Geometry: final body of the model. Coordinates: model frame, mm. Give positions to 0.01 mm unless a question says otherwise; leave off trailing zeros.
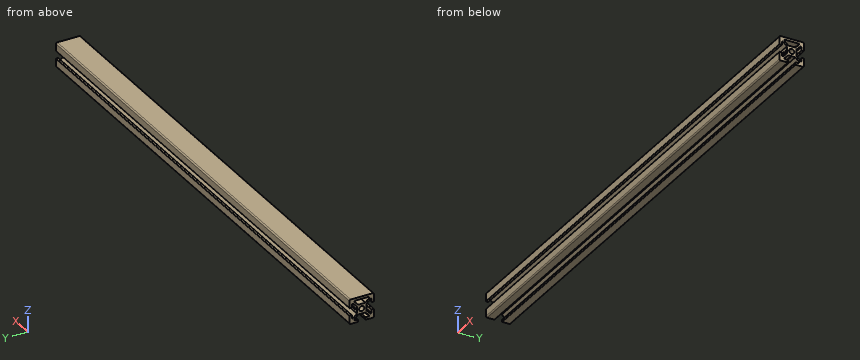
from build123d import *

# Parameters (mm, degrees)
F1_DEPTH = 210


# Not quite as in the source:
# - ends of sketch curves that miss each other by under 0.0002 mm in the source are joined


with BuildPart() as f1:
    # F0 (on Right) → F1 (new body, symmetric)
    with BuildSketch(Plane.YZ):
        with BuildLine():
            Line((9.043565, 10.073321), (0.043565, 10.073321))
            Line((0.043565, 10.073321), (-8.956435, 10.073321))
            ThreePointArc((-8.956435, 10.073321), (-9.6635417812, 9.7804277812), (-9.956435, 9.073321))
            Line((-9.956435, 9.073321), (-9.956435, 3.373321))
            ThreePointArc((-9.956435, 3.373321), (-9.8685670344, 3.1611889656), (-9.656435, 3.073321))
            Line((-9.656435, 3.073321), (-8.256435, 3.073321))
            ThreePointArc((-8.256435, 3.073321), (-8.0443029656, 3.1611889656), (-7.956435, 3.373321))
            Line((-7.956435, 3.373321), (-7.956435, 6.073321))
            Line((-7.956435, 6.073321), (-7.017095, 6.073321))
            Line((-7.017095, 6.073321), (-3.956435, 3.012661))
            Line((-3.956435, 3.012661), (-3.956435, 0.726911))
            ThreePointArc((-3.956435, 0.726911), (-3.9393979324, 0.5975015494), (-3.8894477764, 0.4769111291))
            Line((-3.8894477764, 0.4769111291), (-3.656435, 0.073321))
            Line((-3.656435, 0.073321), (-3.889448, -0.330269))
            ThreePointArc((-3.889448, -0.330269), (-3.956435, -0.580269), (-3.8894477764, -0.8302688709))
            Line((-3.8894477764, -0.8302688709), (-3.707412, -1.145565))
            Line((-3.707412, -1.145565), (-3.956435, -2.426679))
            Line((-3.956435, -2.426679), (-3.956435, -2.866019))
            Line((-3.956435, -2.866019), (-7.017095, -5.926679))
            Line((-7.017095, -5.926679), (-7.956435, -5.926679))
            Line((-7.956435, -5.926679), (-7.956435, -3.226679))
            ThreePointArc((-7.956435, -3.226679), (-8.0443029656, -3.0145469656), (-8.256435, -2.926679))
            Line((-8.256435, -2.926679), (-9.656435, -2.926679))
            ThreePointArc((-9.656435, -2.926679), (-9.8685670344, -3.0145469656), (-9.956435, -3.226679))
            Line((-9.956435, -3.226679), (-9.956435, -8.926679))
            ThreePointArc((-9.956435, -8.926679), (-9.6635417812, -9.6337857812), (-8.956435, -9.926679))
            Line((-8.956435, -9.926679), (-3.256435, -9.926679))
            ThreePointArc((-3.256435, -9.926679), (-3.0443029656, -9.8388110344), (-2.956435, -9.626679))
            Line((-2.956435, -9.626679), (-2.956435, -8.226679))
            ThreePointArc((-2.956435, -8.226679), (-3.0443029656, -8.0145469656), (-3.256435, -7.926679))
            Line((-3.256435, -7.926679), (-5.956435, -7.926679))
            Line((-5.956435, -7.926679), (-5.956435, -6.987339))
            Line((-5.956435, -6.987339), (-2.895775, -3.926679))
            Line((-2.895775, -3.926679), (-0.610025, -3.926679))
            ThreePointArc((-0.610025, -3.926679), (-0.4806155494, -3.9096419324), (-0.3600251291, -3.8596917764))
            Line((-0.3600251291, -3.8596917764), (-0.0645959325, -3.6891257984))
            Line((-0.0645959325, -3.6891257984), (0.2217128734, -3.8544264098))
            ThreePointArc((0.2217128734, -3.8544264098), (0.3921793907, -3.9150473077), (0.5730594828, -3.9110345539))
            ThreePointArc((0.5730594828, -3.9110345539), (0.6346161199, -3.9227524708), (0.697155, -3.926679))
            Line((0.697155, -3.926679), (2.982905, -3.926679))
            Line((2.982905, -3.926679), (6.043565, -6.987339))
            Line((6.043565, -6.987339), (6.043565, -7.926679))
            Line((6.043565, -7.926679), (3.343565, -7.926679))
            ThreePointArc((3.343565, -7.926679), (3.1314329656, -8.0145469656), (3.043565, -8.226679))
            Line((3.043565, -8.226679), (3.043565, -9.626679))
            ThreePointArc((3.043565, -9.626679), (3.1314329656, -9.8388110344), (3.343565, -9.926679))
            Line((3.343565, -9.926679), (9.043565, -9.926679))
            ThreePointArc((9.043565, -9.926679), (9.7506717812, -9.6337857812), (10.043565, -8.926679))
            Line((10.043565, -8.926679), (10.043565, -3.226679))
            ThreePointArc((10.043565, -3.226679), (9.9556970344, -3.0145469656), (9.743565, -2.926679))
            Line((9.743565, -2.926679), (8.343565, -2.926679))
            ThreePointArc((8.343565, -2.926679), (8.1314329656, -3.0145469656), (8.043565, -3.226679))
            Line((8.043565, -3.226679), (8.043565, -5.926679))
            Line((8.043565, -5.926679), (7.104225, -5.926679))
            Line((7.104225, -5.926679), (4.043565, -2.866019))
            Line((4.043565, -2.866019), (4.043565, -2.426679))
            Line((4.043565, -2.426679), (3.794542, -1.145565))
            Line((3.794542, -1.145565), (3.976578, -0.830269))
            ThreePointArc((3.976578, -0.830269), (4.043565, -0.580269), (3.9765777764, -0.3302691291))
            Line((3.9765777764, -0.3302691291), (3.743565, 0.073321))
            Line((3.743565, 0.073321), (3.976578, 0.476911))
            ThreePointArc((3.976578, 0.476911), (4.0265279324, 0.5975015494), (4.043565, 0.726911))
            Line((4.043565, 0.726911), (4.043565, 3.012661))
            Line((4.043565, 3.012661), (7.104225, 6.073321))
            Line((7.104225, 6.073321), (8.043565, 6.073321))
            Line((8.043565, 6.073321), (8.043565, 3.373321))
            ThreePointArc((8.043565, 3.373321), (8.1314329656, 3.1611889656), (8.343565, 3.073321))
            Line((8.343565, 3.073321), (9.743565, 3.073321))
            ThreePointArc((9.743565, 3.073321), (9.9556970344, 3.1611889656), (10.043565, 3.373321))
            Line((10.043565, 3.373321), (10.043565, 9.073321))
            ThreePointArc((10.043565, 9.073321), (9.7506717812, 9.7804277812), (9.043565, 10.073321))
        make_face()
        with BuildLine():
            ThreePointArc((0.043565, 2.173321), (2.143565, 0.073321), (0.043565, -2.026679))
            ThreePointArc((0.043565, -2.026679), (-2.056435, 0.073321), (0.043565, 2.173321))
        make_face(mode=Mode.SUBTRACT)
        with BuildLine():
            Line((2.775798, 4.073321), (0.043565, 4.073321))
            Line((0.043565, 4.073321), (-2.688668, 4.073321))
            ThreePointArc((-2.688668, 4.073321), (-2.8800097162, 4.1113812337), (-3.0422213906, 4.2197676094))
            Line((-3.0422213906, 4.2197676094), (-5.809988, 6.987535))
            ThreePointArc((-5.809988, 6.987535), (-5.9183747663, 7.1497462838), (-5.956435, 7.341088))
            Line((-5.956435, 7.341088), (-5.956435, 7.573321))
            ThreePointArc((-5.956435, 7.573321), (-5.8099883906, 7.9268743906), (-5.456435, 8.073321))
            Line((-5.456435, 8.073321), (0.043565, 8.073321))
            Line((0.043565, 8.073321), (5.543565, 8.073321))
            ThreePointArc((5.543565, 8.073321), (5.8971183906, 7.9268743906), (6.043565, 7.573321))
            Line((6.043565, 7.573321), (6.043565, 7.341088))
            ThreePointArc((6.043565, 7.341088), (6.0055047663, 7.1497462838), (5.8971183906, 6.9875346094))
            Line((5.8971183906, 6.9875346094), (3.129351, 4.219768))
            ThreePointArc((3.129351, 4.219768), (2.9671397162, 4.1113812337), (2.775798, 4.073321))
        make_face(mode=Mode.SUBTRACT)
    extrude(amount=F1_DEPTH, both=True)


solid = f1.part
Item 1: Section query A-A on x = -115. Give the number of separate pieces and of enclosed holes in the cut face, plus the area to 3 significant figures.
Values follow:
separate pieces: 1
enclosed holes: 2
area: 194 mm2
Item 2: Pin query (flat end, axial travel): pin 1 (0.5 mm diameter, centred on x = -27, z = -2.5, fed in from +Y); pin 2 (3 mm diameter, centred on x = 93, y = 0, fed in from -Z). Return the tip coordinate at first contact, or that it passes through.
Values follow:
pin 1: stops at y = 4.04
pin 2: stops at z = -3.93
Item 3: Ray query, probe 1 along Z at (x, y) = (-15.5, 2.5); probe 2 along Z at (x, y) = (31.5, 9); probe 3 along Y at (x, z) = (-192, -8). Return the intervals inside material, ascending.
Values follow:
probe 1: z = -3.93 to 4.07, 8.07 to 10.07
probe 2: z = -9.93 to -2.93, 3.07 to 10.07
probe 3: y = -9.96 to -3.06, 3.15 to 10.04
